Verification items for the finished model (mm, model axes). A direction names the side the tool comes from. Coordinates: 2 decimals unless noted, no trailing zeros. Loops run counter-clockwise (first coordinate to the right, second up) from the corner with the lowest first, then second, coordinate; pieces in that order, holes last.
Q1. Access from +Z, -Z, +X, -X, +Y, -Y to the whole of each face (thin tool, end or side, straight path). Record for faces 5 (the face through (58, -4, 2)), 6 (the face through (-96, 2, 3)), 7 (the face through (58, 4, 2)), 8 (the face through (57.9, -3.5, 4)), 9 (the face through (84.4, -2, 0.4)).
Q2. Mould release check, pull along X, two halves, no side actions. Record for faces 1 (the face through (84.4, 2, 0.4)), 2 (the face through (65, -3, 2)), 3 (the face through (-22, 4, 2)), 4 (the face through (20.8, 2, 0.4)): +X half, -X half, draft (parallel to the pull), parting line (faces both ways), or undercut.
Q3. Material ranges on probe 1 along X at (y, z) = (-5.25, 1.6); probe 2 along X at (y, z) = (-4, 0.85); probe 3 along X at (y, z) = (3.25, 3.7), recorded low to high.
Q4. Sectioned sample at A-A (y = -4). Enter the section's corners in (x, z).
Q5. Sectioned sample at B-B (z = 3.15). Count the separate pieces of the cut face and the enclosed holes in it, then the cut area to 3 significant figures.
Q6. Sectioned sample at C-C (x = -59). Enter the section's corners in (y, z), then the cut area to 3 significant figures.
Q7. Sectioned sample at D-D (x = -15). Enter the section's corners in (y, z).
Q8. Go/stop test with flat-tipped pins: P1, Ø1.2, axis at x = 86, z = 2, coming from the -Y side; P2, Ø0.5, axis at x = 54.5, z = 2, coming from the +Y side; P3, Ø0.8, axis at x = 67.5, z = 3, coming from the -Y side; P4, Ø1.1, axis at y = -1.5, z = 3, coming from the +X side. Record where each tip stops, or that it passes through.
```python
from build123d import *

# Parameters (mm, degrees)
F0_W     = 4
F0_H     = 4
F0_H_2   = 5
F0_W_2   = 76
F0_H_3   = 2.5597222634
F0_H_4   = 2.4402777366
F0_W_3   = 38
F1_DEPTH = 1
F2_W     = 1
F2_H     = 14
F2_H_2   = 5
F3_DEPTH = 3
F4_R     = 4.99999
F2_W_2   = 5
F2_H_3   = 1
F5_DEPTH = 3
F6_R     = 4.99999
F7_DEPTH = 3
F8_R     = 4.99999


# Not quite as in the source:
# - a fillet or chamfer is up to 0.001 mm smaller than in the source, because OpenCascade refuses the exact size


with BuildPart() as f1:
    # F0 (on Top) → F1 (new body)
    with BuildSketch(Plane.XY):
        Polygon((-101, 2), (-97, 2), (-97, 4.5597222634), (-97, 7), (-101, 7), align=None)
        with Locations((-99, 0)):
            Rectangle(F0_W, F0_H)
        with Locations((-99, -4.5)):
            Rectangle(F0_W, F0_H_2)
        with Locations((-59, 0)):
            Rectangle(F0_W_2, F0_H)
        with Locations((-19, 3.2798611317)):
            Rectangle(F0_W, F0_H_3)
        with Locations((-19, 0)):
            Rectangle(F0_W, F0_H)
        with Locations((-19, -4.5)):
            Rectangle(F0_W, F0_H_2)
        with Locations((-19, 5.7798611317)):
            Rectangle(F0_W, F0_H_4)
        with Locations((21, 0)):
            Rectangle(F0_W_2, F0_H)
        with Locations((61, 5.7798611317)):
            Rectangle(F0_W, F0_H_4)
        with Locations((61, 3.2798611317)):
            Rectangle(F0_W, F0_H_3)
        with Locations((61, -4.5)):
            Rectangle(F0_W, F0_H_2)
        with Locations((61, 0)):
            Rectangle(F0_W, F0_H)
        with Locations((82, 0)):
            Rectangle(F0_W_3, F0_H)
    extrude(amount=F1_DEPTH)

    # F2 (on face) → F3 (join)
    with BuildSketch(Plane.XY.offset(1)):
        with Locations((-100.5, 0)):
            Rectangle(F2_W, F2_H)
        with Locations((-97.5, 4.5)):
            Rectangle(F2_W, F2_H_2)
        Polygon((-97, 2), (-98, 2), (-98, 1), (-92, 1), (-92, 2), align=None)
        Polygon((-98, -1), (-98, -2), (-97, -2), (-92, -2), (-92, -1), align=None)
        with Locations((-97.5, -4.5)):
            Rectangle(F2_W, F2_H_2)
    extrude(amount=F3_DEPTH)

    # F4 (radius 5 in the source; OpenCascade refuses exactly that, so slightly less here)
    f4_edges = [f1.edges().sort_by_distance(p)[0] for p in [
        (-97, -2, 2),
        (-98, 1, 2.5),
        (-98, -1, 2.5),
        (-97, 2, 2),
    ]]
    fillet(f4_edges, radius=F4_R)

    # F2 (on face) → F5 (join)
    with BuildSketch(Plane.XY.offset(1)):
        Polygon((-21, 7), (-21, 2), (-21, 1), (-20, 1), (-20, 7), align=None)
        Polygon((-17, 7), (-18, 7), (-18, 1), (-17, 1), (-17, 2), align=None)
        with Locations((-14.5, 1.5)):
            Rectangle(F2_W_2, F2_H_3)
        with Locations((-23.5, 1.5)):
            Rectangle(F2_W_2, F2_H_3)
        with Locations((-23.5, -1.5)):
            Rectangle(F2_W_2, F2_H_3)
        Polygon((-21, -1), (-21, -2), (-21, -7), (-20, -7), (-20, -1), align=None)
        with Locations((-14.5, -1.5)):
            Rectangle(F2_W_2, F2_H_3)
        Polygon((-18, -1), (-18, -7), (-17, -7), (-17, -2), (-17, -1), align=None)
    extrude(amount=F5_DEPTH)

    # F6 (radius 5 in the source; OpenCascade refuses exactly that, so slightly less here)
    f6_edges = [f1.edges().sort_by_distance(p)[0] for p in [
        (-18, 1, 2.5),
        (-20, 1, 2.5),
        (-17, -2, 2),
        (-20, -1, 2.5),
        (-21, -2, 2),
        (-21, 2, 2),
        (-17, 2, 2),
        (-18, -1, 2.5),
    ]]
    fillet(f6_edges, radius=F6_R)

    # F2 (on face) → F7 (join)
    with BuildSketch(Plane.XY.offset(1)):
        Polygon((59, 7), (59, 2), (59, 1), (60, 1), (60, 7), align=None)
        with Locations((65.5, 1.5)):
            Rectangle(F2_W_2, F2_H_3)
        Polygon((63, 7), (62, 7), (62, 1), (63, 1), (63, 2), align=None)
        with Locations((65.5, -1.5)):
            Rectangle(F2_W_2, F2_H_3)
        Polygon((62, -1), (62, -7), (63, -7), (63, -2), (63, -1), align=None)
        with Locations((56.5, 1.5)):
            Rectangle(F2_W_2, F2_H_3)
        with Locations((56.5, -1.5)):
            Rectangle(F2_W_2, F2_H_3)
        Polygon((59, -1), (59, -2), (59, -7), (60, -7), (60, -1), align=None)
    extrude(amount=F7_DEPTH)

    # F8 (radius 5 in the source; OpenCascade refuses exactly that, so slightly less here)
    f8_edges = [f1.edges().sort_by_distance(p)[0] for p in [
        (63, -2, 2),
        (60, 1, 2.5),
        (62, 1, 2.5),
        (60, -1, 2.5),
        (62, -1, 2.5),
        (59, -2, 2),
        (59, 2, 2),
        (63, 2, 2),
    ]]
    fillet(f8_edges, radius=F8_R)


solid = f1.part
```
Geometry check:
1. face 5: +Z, -Z, -Y
1. face 6: +Z
1. face 7: +Z, -Z, +Y
1. face 8: +Z, +X, -X, +Y, -Y
1. face 9: +Z, -Z, +X, -Y
2. face 1: draft
2. face 2: +X half
2. face 3: undercut
2. face 4: undercut
3. probe 1: x = -101 to -100, -97.94 to -96.68, -21.32 to -20.06, -17.94 to -16.68, 58.68 to 59.94, 62.06 to 63.32
3. probe 2: x = -101 to -96, -22 to -16, 58 to 64
3. probe 3: x = -101 to -100, -97.18 to -95.31, -22.69 to -20.82, -17.18 to -15.31, 57.31 to 59.18, 62.82 to 64.69
4. outline: (-101, 0) - (-96, 0) - (-96, 4) - (-97.58, 4) - (-97.58, 1) - (-100, 1) - (-100, 4) - (-101, 4) - close; (-22, 0) - (-16, 0) - (-16, 4) - (-17.58, 4) - (-17.58, 1) - (-20.42, 1) - (-20.42, 4) - (-22, 4) - close; (58, 0) - (64, 0) - (64, 4) - (62.42, 4) - (62.42, 1) - (59.58, 1) - (59.58, 4) - (58, 4) - close
5. separate pieces: 11
5. enclosed holes: 0
5. area: 124 mm2
6. outline: (-2, 0) - (2, 0) - (2, 1) - (-2, 1) - close
6. area: 4.00 mm2
7. outline: (-3, 0) - (3, 0) - (3, 4) - (1.42, 4) - (1.42, 1) - (-1.42, 1) - (-1.42, 4) - (-3, 4) - close
8. P1: passes through
8. P2: stops at y = 2.06
8. P3: stops at y = -2.08
8. P4: stops at x = 68
